For this review, take the finished solid that the model builds, in its own axes (mm). Face numbers are marked on the shaded views. A direction names the side the tool comes from. Give positions to 0.01 mm unless a question says otherwise; leave off trailing zeros. Loops run counter-clockwise (first coordinate to the right, second up) from the corner with the lowest first, then second, coordinate; pieces in that order, holes last. Notation, with made-up numbers: (65.5, 25) - (78.5, 25) arc R17 cw to (78.5, 53) - close; hole circle Ø2 at (-15, 52.5). An arc over 180 degrees is marked (long way). Put each result on its own line as item: value.
from build123d import *

# Parameters (mm, degrees)
F0_W     = 20
F0_H     = 40
F0_R     = 1.75
F1_DEPTH = 5
F2_W     = 20
F2_H     = 30
F2_R     = 3
F3_DEPTH = 5


with BuildPart() as f1:
    # F0 (on Front) → F1 (new body)
    with BuildSketch(Plane.XZ):
        Rectangle(F0_W, F0_H)
        with Locations((-7, 15)):
            Circle(F0_R, mode=Mode.SUBTRACT)
        with Locations((7, 15)):
            Circle(F0_R, mode=Mode.SUBTRACT)
    extrude(amount=F1_DEPTH)

    # F2 (on face) → F3 (join)
    with BuildSketch(Plane(origin=(0, 0, -20), x_dir=(1, 0, 0), z_dir=(0, 0, -1))):
        with Locations((0, -10)):
            Rectangle(F2_W, F2_H)
        with Locations((0, -15)):
            Circle(F2_R, mode=Mode.SUBTRACT)
    extrude(amount=-F3_DEPTH)


solid = f1.part
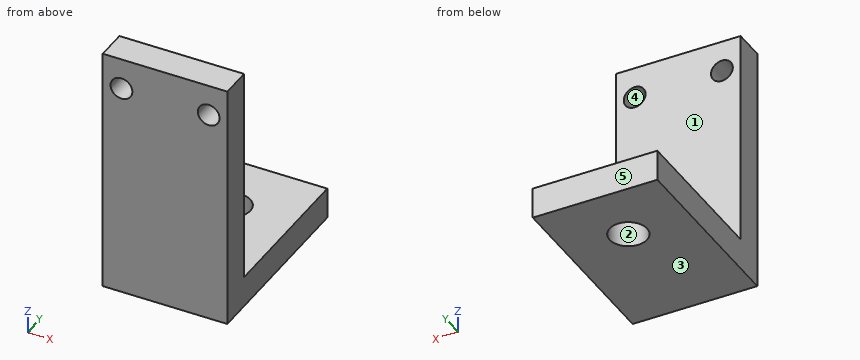
1) Take a section at B-B on z = 15. State the section outline as (x, y) points.
Geometry check:
outline: (-10, -5) - (-8.75, -5) - (-8.75, 0) - (-10, 0) - close; (-5.25, -5) - (5.25, -5) - (5.25, 0) - (-5.25, 0) - close; (8.75, -5) - (10, -5) - (10, 0) - (8.75, 0) - close
2) Insertion check: pin 1 Ø2 at (x, z) = (-1.5, 4.5) entering from +Y; pin 2 Ø1 at (x, y) = (6.5, 2) entering from +Z. Each pin has a flat end and moves straight along its axis. Give the tip position at first contact, or say it passes through.
Geometry check:
pin 1: stops at y = 0
pin 2: stops at z = -15
3) Take a section at A-A on x = 0. State the section outline as (y, z) points.
Geometry check:
outline: (-5, -20) - (12, -20) - (12, -15) - (0, -15) - (0, 20) - (-5, 20) - close; (18, -20) - (25, -20) - (25, -15) - (18, -15) - close
4) For the marked faces 1 and 2, list the 3-axis set-ups (+Z, -Z, +X, -X, +Y, -Y) from which the entire face can be reached by the end or side of a thin tool; tool diameter is ignored.
Geometry check:
face 1: +Z, +X, -X, +Y
face 2: +Z, -Z
5) Take a section at C-C on y = 15.75. State the section outline as (x, z) points.
Geometry check:
outline: (-10, -20) - (-2.9, -20) - (-2.9, -15) - (-10, -15) - close; (2.9, -20) - (10, -20) - (10, -15) - (2.9, -15) - close
6) Draft analysis for pull direction Z (two halves, no side actions). For the marked faces 3, 4 and 5, state which applies: pulls with the +Z half, pulls with the -Z half, needs draft (parallel to the pull), parting line crosses it, or undercut.
Geometry check:
face 3: pulls with the -Z half
face 4: undercut
face 5: needs draft
7) Take a section at D-D on x = 7. State the section outline as (y, z) points.
Geometry check:
outline: (-5, -20) - (25, -20) - (25, -15) - (0, -15) - (0, 13.25) - (-5, 13.25) - close; (-5, 16.75) - (0, 16.75) - (0, 20) - (-5, 20) - close
8) Wall thickness on line 1 (Z direction, x = -7, y = -1.25); line 2 (X direction, y = 15, z = -16.55); line 3 (Y direction, x = 0, z = -16.05): over which ranges is each line inside the solid? List them lowest first.
Geometry check:
line 1: z = -20 to 13.25, 16.75 to 20
line 2: x = -10 to -3, 3 to 10
line 3: y = -5 to 12, 18 to 25
